The listing builds one solid part. Answer for the finished solid, in the listing's coordinates (mm). A direction names the side the tool comes from. Round coordinates to 2 decimals unless told otherwise and drop trailing zeros. Loops run counter-clockwise (first coordinate to the right, second up) from the corner with the lowest first, then second, coordinate; pieces in that order, holes last. Notation, with made-up numbers: M 47,49 L 82,49 A8 cw 82,57 Z; hole C 81,3 d6. An arc over 180 degrees is marked long. Put each result on its own line as item: value. Start each with the question number.
(1) Straight lines are drawn through the part: line 1 (X direction, y = 0.25, z = 3); line 2 (Z direction, x = 28.5, y = -0.25); line 3 (Z direction, x = 24.5, y = 5.5). For each, find the intervals that lie inside material, in ascending order.
(2) Section B-B, the plane y = 0 is taken. Determine the outline of the cut face in (x, z), then the cut area to 3 significant figures.
(3) Section A-A, the plane z = 3.75 is taken. Determine the outline of the cut face in (x, y) (3 decimals), then the cut area to 3 significant figures.
(4) Section C-C, the plane z = -5 is taken. Determine the outline of the cut face in (x, y), then the cut area to 3 significant figures.
(5) Which of the six approach directions +Z, -Z, +X, -X, +Y, -Y give full straight-line access (tool end or side, diameter ignored) to faces 4 (the face through (-36, 0, 5.555)), 5 (the face through (-38.09, -0.1, 2.6)), 6 (the face through (-29.312, 0, 3)), 7 (the face through (28, 0, -0.277))?
(6) Section D-D, the plane y = 4.5 is taken. Determine the outline of the cut face in (x, z), then the cut area to 3 significant figures.
(7) Flat-ended cylindrical pins translate along their axes: P1, Ø4, axis at x = 28.89, y = 0, coming from the +Z side; P2, Ø2, axis at y = 2.5, z = 0.5, coming from the -X side; P3, Ø1.9, axis at y = 2, z = 4.5, coming from the -X side. Find the tip coordinate at first contact, or state that the pin passes through.
(8) Determine the mould class of faces 1 (the face through (22.491, 0, -4)), 2 (the face through (31.92, -0.95, 3)), 3 (the face through (-39.755, 4.822, -3.501)) for opening direction X: released by +X, released by -X, zero draft, split by the parting line, or undercut.
```python
from build123d import *

# Parameters (mm, degrees)
F0_W     = 10.9691135585
F0_H     = 6.3602421433
F1_DEPTH = 6.35
F2_DEPTH = 6.35
F3_R     = 5.08
F5_D     = 6.35
F5_DEPTH = 6.0847096535
F6_R     = 2.2152679596
F7_DEPTH = 12.192


with BuildPart() as f1:
    # F0 (on Front) → F1 (new body)
    with BuildSketch(Plane.XZ):
        Polygon((-29.3124206364, -6.6367746331), (-29.3124206364, -0.2765324898), (-33.8291116059, -0.2765324898), (-37.5162102282, -0.2765324898), (-41.2033051252, -0.2765324898), (-41.2033051252, -6.6367746331), align=None)
        Polygon((22.4912911654, 6.0837096535), (-29.3124206364, 6.0837096535), (-29.3124206364, -0.2765324898), (-29.3124206364, -6.6367746331), (22.4912911654, -6.6367746331), (22.4912911654, -0.2765324898), align=None)
        with Locations((27.9758479446, 2.9035885818)):
            Rectangle(F0_W, F0_H)
    extrude(amount=F1_DEPTH)

    # F2 (add): a face of the model
    f2_faces = [f1.faces().sort_by_distance(p)[0] for p in [
        (-3.6826618353, 0, -0.2997111323),
    ]]
    extrude(f2_faces, amount=F2_DEPTH)

    # F3
    f3_edges = [f1.edges().sort_by_distance(p)[0] for p in [
        (-41.203305, -6.35, -3.456654),
        (-41.203305, 6.35, -3.456654),
        (33.460405, -6.35, 2.903589),
        (33.460405, 6.35, 2.903589),
    ]]
    fillet(f3_edges, radius=F3_R)

    # F5 (through all, one way)
    with BuildSketch(Plane(origin=(0, 0, 0), x_dir=(1, 0, 0), z_dir=(0, 0, -1))):
        with Locations((28.8903526962, 0)):
            Circle(F5_D / 2)
    extrude(amount=-F5_DEPTH, mode=Mode.SUBTRACT)

    # F6 (on face) → F7 (join)
    with BuildSketch(Plane(origin=(0, 0, -6.6367746331), x_dir=(1, 0, 0), z_dir=(0, 0, -1))):
        with Locations((-35.8759947121, 0)):
            Circle(F6_R)
    extrude(amount=-F7_DEPTH)


solid = f1.part
```
Recorded:
1. line 1: x = -38.08 to -33.67, -29.31 to 25.73, 32.06 to 33.46
1. line 2: z = -0.28 to 0
1. line 3: z = -0.28 to 6.08
2. outline: M -41.2,-6.64 L 22.49,-6.64 L 22.49,-0.28 L 33.46,-0.28 L 33.46,6.08 L 32.07,6.08 L 32.07,0 L 25.72,0 L 25.72,6.08 L -29.31,6.08 L -29.31,-0.28 L -33.66,-0.28 L -33.66,5.56 L -38.09,5.56 L -38.09,-0.28 L -41.2,-0.28 Z
2. area: 792 mm²
3. outline: C -35.876,0 d4.431; M -29.312,-6.35 L 28.38,-6.35 A5.08 ccw 33.46,-1.27 L 33.46,1.27 A5.08 ccw 28.38,6.35 L -29.312,6.35 Z; hole C 28.89,0 d6.35
3. area: 770 mm²
4. outline: M -41.2,-1.27 A5.08 ccw -36.12,-6.35 L 22.49,-6.35 L 22.49,6.35 L -36.12,6.35 A5.08 ccw -41.2,1.27 Z
4. area: 798 mm²
5. face 4: +Z, -X, +Y, -Y
5. face 5: +Z
5. face 6: +Z, +Y, -Y
5. face 7: -Z, +X, +Y, -Y
6. outline: M -40.04,-6.64 L 22.49,-6.64 L 22.49,-0.28 L 32.3,-0.28 L 32.3,6.08 L -29.31,6.08 L -29.31,-0.28 L -40.04,-0.28 Z
6. area: 790 mm²
7. P1: stops at z = 0
7. P2: stops at x = -41.17
7. P3: stops at x = -37.83
8. face 1: released by +X
8. face 2: undercut
8. face 3: released by -X
